```python
from build123d import *

# Parameters (mm, degrees)
BOSS_EXTRUDE1_DEPTH = 100
SKETCH3_W           = 80
SKETCH3_H           = 25
BOSS_EXTRUDE2_DEPTH = 100


with BuildPart() as part:
    # Sketch2 → Boss-Extrude1 (new body)
    with BuildSketch(Plane.XY):
        with BuildLine():
            Line((-54.549923262, 1.658687455), (25.450076738, 1.658687455))
            ThreePointArc((25.450076738, 1.658687455), (34.117239254, 29.330582003), (56.685613057, 47.538326449))
            Line((56.685613057, 47.538326449), (56.685613057, 91.538326449))
            Line((56.685613057, 91.538326449), (-40.314386943, 91.538326449))
            Line((-40.314386943, 91.538326449), (-54.549923262, 1.658687455))
        make_face()
    extrude(amount=BOSS_EXTRUDE1_DEPTH)

    # Sketch3 → Boss-Extrude2 (add)
    with BuildSketch(Plane(origin=(0, 0, 0), x_dir=(-1, 0, 0), z_dir=(0, 0, -1))):
        with Locations((-96.685613057, 60.038326449)):
            Rectangle(SKETCH3_W, SKETCH3_H)
    extrude(amount=-BOSS_EXTRUDE2_DEPTH)


solid = part.part
```
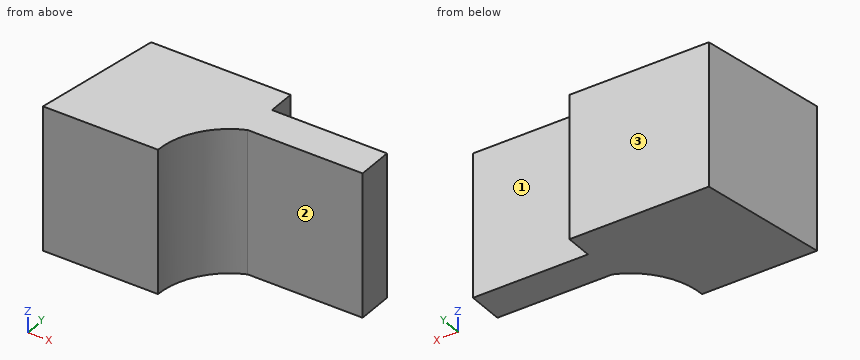
For this review, take the finished solid that the model builds, in its own axes (mm). Face numbers are marked on the shaded views. A direction names the side the tool comes from. Coordinates: 2 decimals unless noted, no trailing zeros. Write each loop counter-clockwise with the first axis right and the second up, starting at its lowest first coordinate (ties: lowest second). Pieces come first, ordered by that corner, then holes.
(1) For pin 1 Ø3 at (y, z) = (22.5, 58.5) entering from -X; pin 2 Ø3 at (x, z) = (59, 85) entering from -Y; pin 3 Ø3 at (y, z) = (45.5, 75.5) entering from -X, all flat-tipped, find the tip position at first contact; note any pin that passes through.
(2) Tool access review of the marked faces 1, 2 and 3: name each direction out of +Z, -Z, +X, -X, +Y, -Y from which nothing blocks a thin tool from reaching the whole face with its end or side.
(3) Add section C-C on y = 76. Give the boundary of the cut face in (x, z), then the cut area to 3 significant figures.
(4) Add section A-A on z = 81. Give the boundary of the cut face in (x, y).
(5) Add section B-B on x = 108. Give the boundary of the cut face in (y, z).
(6) Wall thickness on probe 1 along Y at (x, z) = (79.5, 40.5); probe 2 along X at (y, z) = (70.5, 18); probe 3 along X at (y, z) = (69.5, 17): over which ranges is each line inside the solid? List them lowest first.
Answer sheet:
1. pin 1: stops at x = -51.49
1. pin 2: stops at y = 47.54
1. pin 3: stops at x = -47.84
2. face 1: +Z, -Z, +X, +Y
2. face 2: +Z, -Z, +X, -Y
2. face 3: +Z, -Z, +X, -X, +Y
3. outline: (-42.78, 0) - (56.69, 0) - (56.69, 100) - (-42.78, 100) - close
3. area: 9,950 mm2
4. outline: (-54.55, 1.66) - (25.45, 1.66) arc R50 cw to (56.69, 47.54) - (136.69, 47.54) - (136.69, 72.54) - (56.69, 72.54) - (56.69, 91.54) - (-40.31, 91.54) - close
5. outline: (47.54, 0) - (72.54, 0) - (72.54, 100) - (47.54, 100) - close
6. probe 1: y = 47.54 to 72.54
6. probe 2: x = -43.65 to 136.69
6. probe 3: x = -43.8 to 136.69
